from build123d import *

# Parameters (mm, degrees)
SKETCH2_R           = 6.35
BOSS_EXTRUDE1_DEPTH = 12.7
BOSS_EXTRUDE2_REACH = 91.803
SKETCH4_R           = 7.62


with BuildPart() as part:
    # Sketch2 → Boss-Extrude1 (new body)
    with BuildSketch(Plane(origin=(0, 0, 0), x_dir=(1, 0, 0), z_dir=(0, 1, 0))):
        with BuildLine():
            Line((-63.5, 101.6), (-38.1, 101.6))
            Line((-38.1, 101.6), (-38.1, 88.9))
            ThreePointArc((-38.1, 88.9), (-31.75, 82.55), (-25.4, 88.9))
            Line((-25.4, 88.9), (-25.4, 101.6))
            Line((-25.4, 101.6), (0, 101.6))
            ThreePointArc((0, 101.6), (12.7, 88.9), (0, 76.2))
            Line((0, 76.2), (-12.7, 76.2))
            Line((-12.7, 76.2), (-12.7, 12.7))
            Line((-12.7, 12.7), (0, 12.7))
            ThreePointArc((0, 12.7), (12.7, 0), (0, -12.7))
            Line((0, -12.7), (-63.5, -12.7))
            ThreePointArc((-63.5, -12.7), (-76.2, 0), (-63.5, 12.7))
            Line((-63.5, 12.7), (-50.8, 12.7))
            Line((-50.8, 12.7), (-50.8, 76.2))
            Line((-50.8, 76.2), (-63.5, 76.2))
            ThreePointArc((-63.5, 76.2), (-76.2, 88.9), (-63.5, 101.6))
        make_face()
        Circle(SKETCH2_R, mode=Mode.SUBTRACT)
        with Locations((0, 88.9)):
            Circle(SKETCH2_R, mode=Mode.SUBTRACT)
        with Locations((-63.5, 0)):
            Circle(SKETCH2_R, mode=Mode.SUBTRACT)
        with Locations((-63.5, 88.9)):
            Circle(SKETCH2_R, mode=Mode.SUBTRACT)
    extrude(amount=BOSS_EXTRUDE1_DEPTH)

    # Sketch4 → Boss-Extrude2 (add, up to next)
    with BuildSketch(Plane(origin=(0, 12.7, 12.7), x_dir=(1, 0, 0), z_dir=(0, 0.707106781, 0.707106781)), mode=Mode.PRIVATE) as boss_extrude2_sk1:
        with BuildLine():
            Line((-50.8, 0), (-50.8, 35.052))
            ThreePointArc((-50.8, 35.052), (-31.75, 54.102), (-12.7, 35.052))
            Line((-12.7, 35.052), (-12.7, 0))
            Line((-12.7, 0), (-50.8, 0))
        make_face()
        with Locations((-31.75, 35.052)):
            Circle(SKETCH4_R, mode=Mode.SUBTRACT)
    boss_extrude2_tool1 = extrude(boss_extrude2_sk1.sketch, amount=-BOSS_EXTRUDE2_REACH, mode=Mode.PRIVATE) - part.part
    add(boss_extrude2_tool1.solids().sort_by_distance((-31.75, 29.771946, -4.371946))[0])


solid = part.part
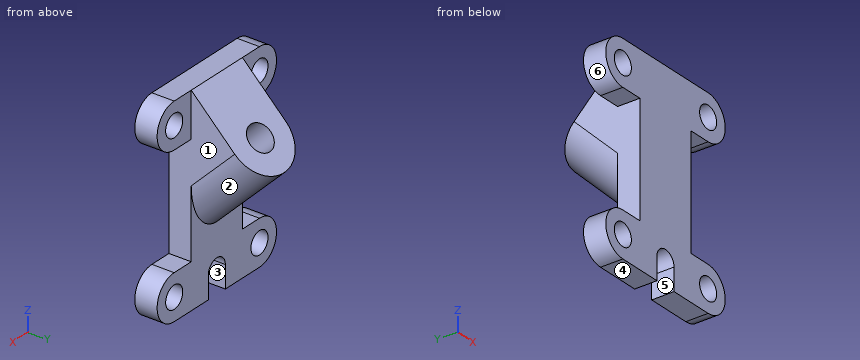
Input: part model. Units: mm. Frame: model coordinates. Face numbers are marked on the shaded views. A direction names the side the tool comes from. Give positions to 0.01 mm unless a question says otherwise; leave off trailing zeros. Loops run counter-clockwise (first coordinate to the right, second up) from the corner with the lowest first, then second, coordinate; pieces in that order, holes last. Notation, with made-up numbers: M 25.25,47.25 L 45.25,47.25 A20 ccw 45.25,84.25 Z; hole C -13.75,27.5 d11. An arc over 180 degrees is marked long. Use one line per item in the form item = value.
1. Section query C-C, the plane x = -19. Return the cut outline in (y, z).
Numbers:
outline = M 0,-101.6 L 12.7,-101.6 L 12.7,-56.89 L 47.49,-22.09 L 12.7,12.7 L 0,12.7 Z
2. Section query A-A, the plane z = 0. Return the cut outline in (x, y), and give its area (3 significant figures).
Numbers:
outline = M -76.2,0 L -69.85,0 L -69.85,12.7 L -76.2,12.7 Z; M -57.15,0 L -6.35,0 L -6.35,12.7 L -12.7,12.7 L -12.7,25.4 L -50.8,25.4 L -50.8,12.7 L -57.15,12.7 Z; M 6.35,0 L 12.7,0 L 12.7,12.7 L 6.35,12.7 Z
area = 1,290 mm²
3. First-contact query: pin 1 (10 mm diameter, centred on x = -63.5, y = 21.5, fed in from -Z); pin 2 (4 mm diameter, centred on x = -29.5, y = 36.5, fed in from +Z); pin 3 (5 mm diameter, centred on y = 9, z = -66, fed in from -X); pin 4 (16.5 mm diameter, centred on x = 0, z = -88.9, fed in from +Y). Flat tips, straight axial feed; report the tip coordinate or a pass-through.
Numbers:
pin_1 = through
pin_2 = -21.08
pin_3 = -50.8
pin_4 = 12.7
4. Section query B-B, the plane x = -31.75. Return the cut outline in (y, z).
Numbers:
outline = M 0,-82.55 L 12.7,-82.55 L 12.7,-63.81 L 50.96,-25.56 L 42.87,-17.47 L 12.7,-47.65 L 12.7,-26.09 L 32.1,-6.7 L 12.7,12.7 L 0,12.7 Z
5. Reachability of the marked faces 1, 2 and 3 from +Z, -Z, +X, -X, +Y, -Y: full face, straight path, thin tool, end or side. Return the list, or none.
Numbers:
face_1 = +X, +Y
face_2 = -Z, +Y
face_3 = -Z, +Y, -Y
6. Line query: L1, parallel to X at y = 10, z = 0; L2, parallel to X at y = 9, z = -88.5; L3, parallel to Z at x = -63.5, y = 3. Output: solid intervals per line, ascending.
Numbers:
L1 = -76.2 to -69.85, -57.15 to -6.35, 6.35 to 12.7
L2 = -76.19 to -69.84, -57.16 to -38.09, -25.41 to -6.34, 6.34 to 12.69
L3 = -101.6 to -95.25, -82.55 to -76.2, -12.7 to -6.35, 6.35 to 12.7
7. Pull-direction query (Z, two-part tool) for the marked faces 4, 5 and 6; classes: released by +Z, released by -Z, zero draft, split by the parting line, or undercut.
Numbers:
face_4 = released by -Z
face_5 = zero draft
face_6 = undercut
